Can you work these out from the drawing? Everything is in mm from the part's minimum corner. A direction names the side the tool comes from. Coordinates: 2 decimals unless noted, no trailing zeros. Loops run counter-clockwise (first coordinate to the right, second up) from the corner with the lowest first, then second, coordinate; pieces in that order, holes last. Notation, with made-up numbers: M 30.5,0 L 73.5,0 A8 ccw 73.5,9 Z; hole C 81.25,4 d10. An arc over 180 degrees is marked long. Write each question's results on one line, items separated by ' | '.
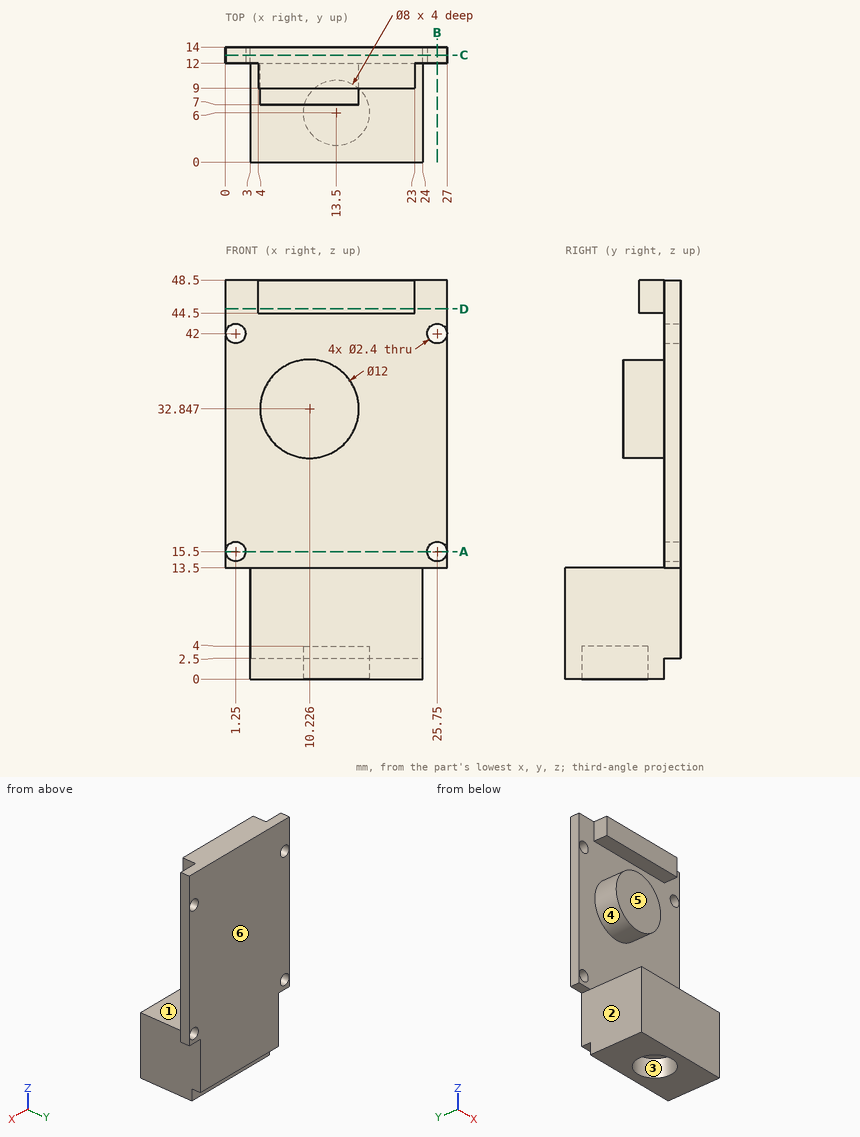
(1) If we mould it in two halves opening along X, with no side actions, what happens to the marked faces 1, 2 and 3? For each: released by +X, released by -X, zero draft, split by the parting line, or undercut.
Reported:
face 1: zero draft | face 2: released by -X | face 3: undercut
(2) Which directions (+Z, -Z, +X, -X, +Y, -Y) give clear straight access to the entire face, cutting with the end or side of a thin tool? Please do the marked faces 4, 5 and 6.
Reported:
face 4: -Y | face 5: +Z, +X, -X, -Y | face 6: +Z, -Z, +X, -X, +Y
(3) Imagine slicing it at D-D, the plane z = 45. List the corners of the cut face in (x, y) for me.
Reported:
outline: M 0,12 L 4,12 L 4,9 L 23,9 L 23,12 L 27,12 L 27,14 L 0,14 Z
(4) Imagine slicing it at A-A, the plane z = 15.5. List the corners of the cut face in (x, y) for me.
Reported:
outline: M 0,12 L 0.05,12 L 0.05,14 L 0,14 Z; M 2.45,12 L 24.55,12 L 24.55,14 L 2.45,14 Z; M 26.95,12 L 27,12 L 27,14 L 26.95,14 Z
(5) Imagine slicing it at B-B, the plane x = 25.75. List the corners of the cut face in (y, z) for me.
Reported:
outline: M 12,13.5 L 14,13.5 L 14,14.3 L 12,14.3 Z; M 12,16.7 L 14,16.7 L 14,40.8 L 12,40.8 Z; M 12,43.2 L 14,43.2 L 14,48.5 L 12,48.5 Z
(6) Imagine slicing it at C-C, the plane y = 13. List the corners of the cut face in (x, z) for me.
Reported:
outline: M 0,13.5 L 3,13.5 L 3,2.5 L 24,2.5 L 24,13.5 L 27,13.5 L 27,48.5 L 0,48.5 Z; hole C 1.25,15.5 d2.4; hole C 1.25,42 d2.4; hole C 25.75,15.5 d2.4; hole C 25.75,42 d2.4
(7) Please list where these lines run through material, in increasing order: probe 1 along Z at (x, y) = (1.25, 12.8); probe 2 along Z at (x, y) = (10, 10.75); probe 3 along Y at (x, z) = (6.25, 37). Write a range as from..to.
Reported:
probe 1: z = 13.5..14.3, 16.7..40.8, 43.2..48.5 | probe 2: z = 0..13.5, 26.85..38.84, 44.5..48.5 | probe 3: y = 7..14
(8) Will these pins go through, and if not, where does the flat tip stop? P1, Ø1.5, axis at x = 23, y = 6.5, coming from the +Z side; P2, Ø4, axis at y = 10, z = 9, coming from the +X side; P3, Ø3.5, axis at x = 8.5, z = 35.5, coming from the -Y side.
Reported:
P1: stops at z = 13.5 | P2: stops at x = 24 | P3: stops at y = 7
